Autodesk Inventor part; units mm, degrees
ref_plane "XZ Plane" through (0, 0, 0) normal (0, 1, 0) x (-1, 0, 0)
ref_plane "XY Plane" through (0, 0, 0) normal (0, 0, 1) x (1, 0, 0)
sketch "Sketch1" plane through (0, 0, 0) normal (0, 1, 0) x (-1, 0, 0)
  circle A0 centre (0, 0) radius 19
  circle A1 centre (0, 0) radius 18
  dimension "d0" = 38
  dimension "d1" = 36
extrude "Extrusion1" add sketch "Sketch1" along normal blind 3
ref_plane "Work Plane1" through (19, 0, 0) normal (1, 0, 0) x (0, 1, 0)
sketch "Sketch2" plane through (19, 0, 0) normal (1, 0, 0) x (0, 1, 0)
  line L0 (0, 1) -> (5, 1)
  line L1 (5, 1) -> (5, -1)
  line L2 (5, -1) -> (0, -1)
  line L3 (0, -1) -> (0, 1)
  point P0 (0, 0)
  dimension "d4" = 1
  dimension "d5" = 1
  dimension "d6" = 0
  dimension "d7" = 5
extrude "Extrusion2" cut sketch "Sketch2" against normal blind 5
properties part number "ringLoop" material "Copper"
The model under review builds one solid part; all positions refer to its coordinate system, in mm. Round coordinates to 2 decimals unless told otherwise and drop trailing zeros. Loops run counter-clockwise (first coordinate to the right, second up) from the corner with the lowest first, then second, coordinate; pieces in that order, holes last. Notation, with made-up numbers: M 19.25,79.5 L 54.25,79.5 A31 ccw 54.25,116.5 Z; hole C 13.25,89.5 d2. An arc over 180 degrees is marked long. Put each result on its own line as item: value.
Q1. Mouldability with a two-part tool opening along Z and no side actions: class faces 1 (the flat face through (18.5, 1.5, -1)), 2 (the flat face through (-7, 0, 17)), 3 (the flat face through (18.5, 1.5, 1)) as released by +Z, released by -Z, zero draft, split by the parting line, or undercut.
Result set:
face 1: undercut
face 2: zero draft
face 3: undercut
Q2. Consider section B-B, the plane z = -14. Give the boundary of the cut face in (x, y).
Result set:
outline: M -12.85,0 L -11.31,0 L -11.31,3 L -12.85,3 Z; M 11.31,0 L 12.85,0 L 12.85,3 L 11.31,3 Z
Q3. Consider section C-C, the plane y = 1.65. Give the boundary of the cut face in (x, z), then the cut area to 3 significant figures.
Result set:
outline: M 17.97,-1 A18 cw long 17.97,1 L 18.97,1 A19 ccw long 18.97,-1 Z
area: 114 mm²
Q4. To check wall thickness, follow L1, parallel to Z at x = 11, y = 1.8; L2, parallel to Z at x = 13.5, y = 2.9; L3, parallel to X at y = 2.25, z = 6.5. State the ranges of each line that lie inside material, in increasing order.
Result set:
L1: z = -15.49 to -14.25, 14.25 to 15.49
L2: z = -13.37 to -11.91, 11.91 to 13.37
L3: x = -17.85 to -16.79, 16.79 to 17.85
Q5. Consider section A-A, the plane x = -12. Give the boundary of the cut face in (y, z).
Result set:
outline: M 0,-14.73 L 3,-14.73 L 3,-13.42 L 0,-13.42 Z; M 0,13.42 L 3,13.42 L 3,14.73 L 0,14.73 Z
